from build123d import *

# Parameters (mm, degrees)
CROQUIS1_W              = 32.5
CROQUIS1_H              = 21
SALIENTE_EXTRUIR1_DEPTH = 16
CROQUIS2_R              = 2
SALIENTE_EXTRUIR2_DEPTH = 15
CROQUIS3_R              = 3
SALIENTE_EXTRUIR3_DEPTH = 1.5
REDONDEO1_R             = 1.7


with BuildPart() as part:
    # Croquis1 → Saliente-Extruir1 (new body)
    with BuildSketch(Plane(origin=(0, 0, 0), x_dir=(1, 0, 0), z_dir=(0, 1, 0))):
        Rectangle(CROQUIS1_W, CROQUIS1_H)
    extrude(amount=SALIENTE_EXTRUIR1_DEPTH)

    # Croquis2 → Saliente-Extruir2 (add)
    with BuildSketch(Plane(origin=(0, 16, 0), x_dir=(1, 0, 0), z_dir=(0, 1, 0))):
        with Locations((-9, 0)):
            Circle(CROQUIS2_R)
        with Locations((9, 0)):
            Circle(CROQUIS2_R)
    extrude(amount=SALIENTE_EXTRUIR2_DEPTH)

    # Croquis3 → Saliente-Extruir3 (add)
    with BuildSketch(Plane.XZ):
        Polygon((-16.25, 8.754302239), (-25.5, 6), (-25.5, -6), (-16.25, -8.754302239), align=None)
        with Locations((-20, 0)):
            Circle(CROQUIS3_R, mode=Mode.SUBTRACT)
        Polygon((16.25, -8.754302239), (25.5, -6), (25.5, 6), (16.25, 8.754302239), align=None)
        with Locations((20, 0)):
            Circle(CROQUIS3_R, mode=Mode.SUBTRACT)
    extrude(amount=-SALIENTE_EXTRUIR3_DEPTH)

    # Redondeo1
    redondeo1_edges = [part.edges().sort_by_distance(p)[0] for p in [
        (0, 0, 10.5),
        (0, 0, -10.5),
        (16.25, 8, 10.5),
        (-16.25, 8, 10.5),
        (-16.25, 8, -10.5),
        (16.25, 8, -10.5),
    ]]
    fillet(redondeo1_edges, radius=REDONDEO1_R)


solid = part.part
Build history of the part. All positions in model axes, mm. A direction names the side the tool comes from. Coordinates: 2 decimals unless noted, no trailing zeros. Order: outer loops, then holes, each group sorted by start corner. A loop starts at its lowest first (then second) coordinate and runs counter-clockwise, first axis right, second up. Notation, with made-up numbers: (2.25, 18.25) -> (58.25, 18.25) arc R31 ccw to (58.25, 57.25) -> close; hole circle Ø11 at (44.5, 89). An arc over 180 degrees is marked (long way). One line per item, written item: value.
(1) Probe line 1 (Y direction, x = 18, z = -3.5); line 2 (Y direction, x = -1.5, z = 0.5); line 3 (X direction, y = 25.5, z = 1.25). List the from-to ranges inside material, lowest first. Write a range as [from, to].
Checked values:
line 1: [0, 1.5]
line 2: [0, 16]
line 3: [-10.56, -7.44], [7.44, 10.56]
(2) Drop flat-ended pins along their axis: pin 1 Ø6 at (y, z) = (13, 7.5) entering from +X; pin 2 Ø4.5 at (x, z) = (21, 2) entering from +Y; pin 3 Ø8 at (y, z) = (8.5, -6) entering from -X. Give the stop position or say it passes through.
Checked values:
pin 1: x = 16.25
pin 2: y = 1.5
pin 3: x = -16.25
(3) Tool access for faces 5 (the cylindrical face through (-10.6, 23.4, 1.2)), 6 (the flat face through (-23, 1.5, -2)), 7 (the flat face through (23, 1.5, -2)): list every direction of +Z, -Z, +X, -X, +Y, -Y with a clear straight run to the whole face (end or side of a thin tool).
Checked values:
face 5: +Y
face 6: +Z, -Z, -X, +Y
face 7: +Z, -Z, +X, +Y
(4) Slice it at D-D, the plane x = -20. List the corners of the cut face in (y, z).
Checked values:
outline: (0, -7.64) -> (1.5, -7.64) -> (1.5, -3) -> (0, -3) -> close; (0, 3) -> (1.5, 3) -> (1.5, 7.64) -> (0, 7.64) -> close
(5) Slice it at C-C, the plane y = 27. List the corners of the cut face in (x, z).
Checked values:
outline: circle Ø4 at (-9, 0); circle Ø4 at (9, 0)
(6) Mould opens along X. For faces 1 (the cylindrical face through (-23, 1, 0)), 2 (the flat face through (0, 9, -10.5)), 3 (the cylindrical face through (7, 23, 0)), 4 (the flat face through (16.25, 8, 0)) say: pulls with the +X half, pulls with the -X half, needs draft (parallel to the pull), parting line crosses it, or undercut.
Checked values:
face 1: undercut
face 2: needs draft
face 3: undercut
face 4: pulls with the +X half
(7) Slice it at A-A, the plane z = 0. List the corners of the cut face in (x, y), plus the area to 3 significant figures.
Checked values:
outline: (-25.5, 0) -> (-23, 0) -> (-23, 1.5) -> (-25.5, 1.5) -> close; (-17, 0) -> (17, 0) -> (17, 1.5) -> (16.25, 1.5) -> (16.25, 16) -> (11, 16) -> (11, 31) -> (7, 31) -> (7, 16) -> (-7, 16) -> (-7, 31) -> (-11, 31) -> (-11, 16) -> (-16.25, 16) -> (-16.25, 1.5) -> (-17, 1.5) -> close; (23, 0) -> (25.5, 0) -> (25.5, 1.5) -> (23, 1.5) -> close
area: 650 mm2
(8) Slice it at B-B, the plane x = 9. List the corners of the cut face in (y, z), plus the area to 3 significant figures.
Checked values:
outline: (0, -8.8) arc R1.7 ccw to (1.7, -10.5) -> (16, -10.5) -> (16, -2) -> (31, -2) -> (31, 2) -> (16, 2) -> (16, 10.5) -> (1.7, 10.5) arc R1.7 ccw to (0, 8.8) -> close
area: 395 mm2
